Can you work these out from the drawing? Everything is in mm from the part's minimum corner. A direction names the side the tool comes from. Coordinates: 2 decimals unless noted, no trailing zeros. Order: outer loops, then holes, each group sorted by start corner. A loop starts at its lowest first (then second) coordinate and runs counter-clockwise, first axis right, second up. Notation, with made-up numbers: M 24,87.5 L 83,87.5 A29 ccw 83,126.5 Z; hole C -6,37.5 d2. An arc over 180 degrees is marked long. Answer as CSV lines item,"result". Start each with the question number.
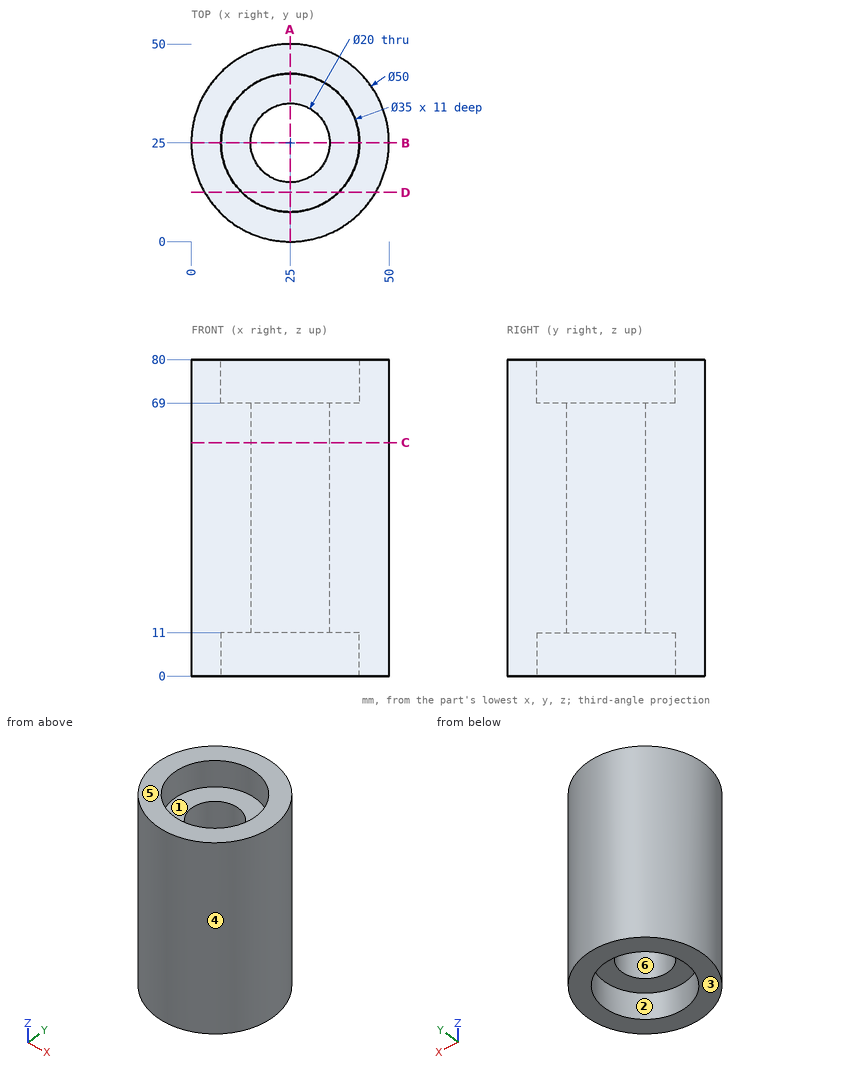
1) Suppose I cut it at D-D on y = 12.5. Please give me the cut outline in (x, z), plus the area to 3 significant figures.
2) Suppose I cut it at A-A on x = 25. Please give me the cut outline in (y, z), plus the area to 3 significant figures.
3) Will these pins go through, and if not, where does the flat tip stop? pin 1 Ø12 at (x, y) = (25, 25) entering from -Z; pin 2 Ø10 at (x, z) = (23, 45.5) entering from +Y; pin 3 Ø1.5 at (y, z) = (12.5, 30) entering from -X; pin 4 Ø6 at (x, z) = (33, 25) entering from +Y.
4) If we mould it in two halves opening along Y, with no side actions, what happens to the marked faces 4, 5 and 6? For each: released by +Y, released by -Y, zero draft, split by the parting line, or undercut.
5) Which directions (+Z, -Z, +X, -X, +Y, -Y) give clear straight access to the entire face, cutting with the end or side of a thin tool? Please do the marked faces 1, 2 and 3.
6) Suppose I cut it at C-C on z = 59. Please give me the cut outline in (x, y), plus the area to 3 significant figures.
7) I need wall thicknesses on line 1 (Y direction, x = 25, z = 7.25); line 2 (Y direction, x = 25, z = 28.5); line 3 (Z direction, x = 25.5, y = 12.5). Which ranges of each line are inside material? Lowest first, please. Write a range as [from, to].
Output:
1,outline,"M 3.35,0 L 12.75,0 L 12.75,11 L 37.25,11 L 37.25,0 L 46.65,0 L 46.65,80 L 37.25,80 L 37.25,69 L 12.75,69 L 12.75,80 L 3.35,80 Z"
1,area,"2,930 mm²"
2,outline,"M 0,0 L 7.5,0 L 7.5,11 L 15,11 L 15,69 L 7.5,69 L 7.5,80 L 0,80 Z; M 35,11 L 42.5,11 L 42.5,0 L 50,0 L 50,80 L 42.5,80 L 42.5,69 L 35,69 Z"
2,area,"2,070 mm²"
3,pin 1,"through"
3,pin 2,"y = 50"
3,pin 3,"x = 2.93"
3,pin 4,"y = 49.49"
4,face 4,"split by the parting line"
4,face 5,"zero draft"
4,face 6,"undercut"
5,face 1,"+Z"
5,face 2,"-Z"
5,face 3,"-Z, +X, -X, +Y, -Y"
6,outline,"C 25,25 d50; hole C 25,25 d20"
6,area,"1,650 mm²"
7,line 1,"[0, 7.5], [42.5, 50]"
7,line 2,"[0, 15], [35, 50]"
7,line 3,"[11, 69]"
